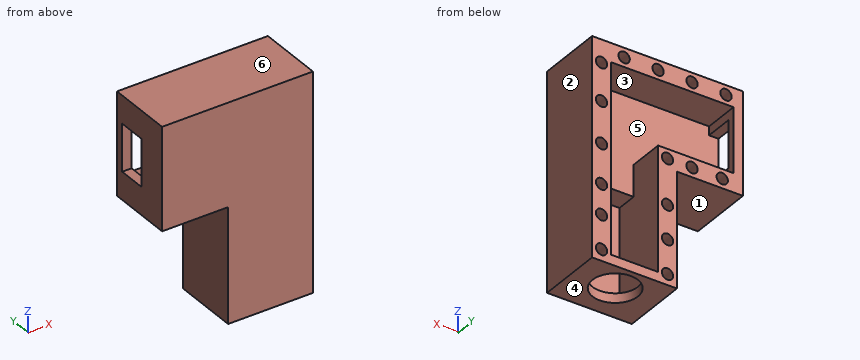
```python
from build123d import *

# Parameters (mm, degrees)
EXTRUDE_1_DEPTH     = 35
EXTRUDE_2_DEPTH     = 5
SKETCH_4_R          = 3
CUT_EXTRUDE_1_DEPTH = 20
SKETCH_6_W          = 25
SKETCH_6_H          = 16.678910785
EXTRUDE_3_DEPTH     = 11
SKETCH_7_W          = 65
SKETCH_7_H          = 34.285714286
EXTRUDE_4_DEPTH     = 11
SKETCH_8_R          = 12.052464441
CUT_EXTRUDE_2_DEPTH = 11
SKETCH_9_W          = 25
SKETCH_9_H          = 15
CUT_EXTRUDE_3_DEPTH = 11


with BuildPart() as part:
    # Эскиз1 → Бобышка-Вытянуть1 (new body)
    with BuildSketch(Plane(origin=(0, 0, 0), x_dir=(1, 0, 0), z_dir=(0, 1, 0))):
        Polygon((-25.991917961, 25.824175824), (0, 25.824175824), (0, 86.538461538), (45, 86.538461538), (45, -28.461538462), (-35, -28.461538462), (-35, 25.824175824), align=None)
        Polygon((-30, -18.461538462), (35, -18.461538462), (35, 21.538461538), (35, 81.538461538), (10, 81.538461538), (10, 15.824175824), (-30, 15.824175824), align=None, mode=Mode.SUBTRACT)
    extrude(amount=EXTRUDE_1_DEPTH)

    # Эскиз3 → Бобышка-Вытянуть2 (add)
    with BuildSketch(Plane.XZ):
        Polygon((35, -81.538461538), (35, 18.461538462), (-30, 18.461538462), (-30, -15.824175824), (10, -15.824175824), (10, -81.538461538), align=None)
    extrude(amount=-EXTRUDE_2_DEPTH)

    # Эскиз4 → Вырез-Вытянуть1 (cut)
    with BuildSketch(Plane(origin=(0, 35, 0), x_dir=(1, 0, 0), z_dir=(0, 1, 0))):
        with Locations(Location((40, 80.538461538, 0), (0, 0, 270))):
            Circle(SKETCH_4_R)
        with Locations(Location((40, 62.538461538, 0), (0, 0, 270))):
            Circle(SKETCH_4_R)
        with Locations(Location((40, 46.538461538, 0), (0, 0, 270))):
            Circle(SKETCH_4_R)
        with Locations(Location((40, 25.538461538, 0), (0, 0, 270))):
            Circle(SKETCH_4_R)
        with Locations(Location((40, 3.538461538, 0), (0, 0, 270))):
            Circle(SKETCH_4_R)
        with Locations(Location((40, -16.461538462, 0), (0, 0, 270))):
            Circle(SKETCH_4_R)
        with Locations(Location((5, 80.824175824, 0), (0, 0, 270))):
            Circle(SKETCH_4_R)
        with Locations(Location((5, 62.824175824, 0), (0, 0, 270))):
            Circle(SKETCH_4_R)
        with Locations(Location((5, 44.824175824, 0), (0, 0, 270))):
            Circle(SKETCH_4_R)
        with Locations(Location((-24, 20.824175824, 0), (0, 0, 270))):
            Circle(SKETCH_4_R)
        with Locations(Location((-8, 20.824175824, 0), (0, 0, 270))):
            Circle(SKETCH_4_R)
        with Locations(Location((5, 20.824175824, 0), (0, 0, 270))):
            Circle(SKETCH_4_R)
        with Locations(Location((-26, -23.461538462, 0), (0, 0, 270))):
            Circle(SKETCH_4_R)
        with Locations(Location((-8, -23.461538462, 0), (0, 0, 270))):
            Circle(SKETCH_4_R)
        with Locations(Location((10, -23.461538462, 0), (0, 0, 270))):
            Circle(SKETCH_4_R)
        with Locations(Location((28, -23.461538462, 0), (0, 0, 270))):
            Circle(SKETCH_4_R)
    extrude(amount=-CUT_EXTRUDE_1_DEPTH, mode=Mode.SUBTRACT)

    # Эскиз6 → Бобышка-Вытянуть3 (add)
    with BuildSketch(Plane(origin=(0, 5, 0), x_dir=(1, 0, 0), z_dir=(0, 1, 0))):
        with Locations((22.5, 24.163631217)):
            Rectangle(SKETCH_6_W, SKETCH_6_H)
    extrude(amount=EXTRUDE_3_DEPTH)

    # Эскиз7 → Бобышка-Вытянуть4 (add)
    with BuildSketch(Plane(origin=(0, 5, 0), x_dir=(1, 0, 0), z_dir=(0, 1, 0))):
        with Locations((2.5, -1.318681319)):
            Rectangle(SKETCH_7_W, SKETCH_7_H)
    extrude(amount=EXTRUDE_4_DEPTH)

    # Эскиз8 → Вырез-Вытянуть2 (cut)
    with BuildSketch(Plane.XY.offset(-81.538461538)):
        with Locations((22.5, 20)):
            Circle(SKETCH_8_R)
    extrude(amount=-CUT_EXTRUDE_2_DEPTH, mode=Mode.SUBTRACT)

    # Эскиз9 → Вырез-Вытянуть3 (cut)
    with BuildSketch(Plane(origin=(-30, 0, 0), x_dir=(0, 0, -1), z_dir=(1, 0, 0))):
        with Locations((-1.318681319, 23.5)):
            Rectangle(SKETCH_9_W, SKETCH_9_H)
    extrude(amount=-CUT_EXTRUDE_3_DEPTH, mode=Mode.SUBTRACT)


solid = part.part
```
Here's how the part is built. I have some questions about the finished solid (model axes, mm). Face numbers are marked on the shaded views. A direction names the side the tool comes from. Give positions to 0.01 mm unless a question says otherwise; leave off trailing zeros. Order: outer loops, then holes, each group sorted by start corner. A loop starts at its lowest first (then second) coordinate and runs counter-clockwise, first axis right, second up. Notation, with made-up numbers: (39, -7.5) - (86, -7.5) arc R30 cw to (86, 25.5) - close; hole circle Ø9 at (-28.5, -29). An arc over 180 degrees is marked (long way). Answer as a JSON object with one key per item and string values. Group by question number.
Item 1: For P1, Ø5.5, axis at x = -26, z = 23.46, coming from the +Y side; P2, Ø5, axis at x = -26, y = 22, coming from the -Z side, each with a flat end and sliding along its axis, tell me the tip position at first contact or that it passes through.
Item 2: If we section it at B-B on z = -13.5: Please give me the cut outline in (x, y).
Item 3: If we section it at D-D on x = -8: Please give me the cut outline in (y, z), and give its area (3 significant figures).
Item 4: Which directions (+Z, -Z, +X, -X, +Y, -Y) give clear straight access to the entire face, cutting with the end or side of a thin tool? Please do the marked faces 1, 2 and 3.
Item 5: Please list where these lines run through material, in increasing order: probe 1 along X at (y, z) = (26, -74.5); probe 2 along Z at (x, y) = (-18, 12); probe 3 along Z at (x, y) = (15.5, 22).
Item 6: If we section it at A-A on x = 22.5: Please give me the cut outline in (y, z), and give its area (3 significant figures).
Item 7: If we mould it in two halves opening along Z, with no side actions, what happens to the marked faces 4, 5 and 6? For each: pulls with the +Z half, pulls with the -Z half, needs draft (parallel to the pull), parting line crosses it, or undercut.
Item 8: If we section it at C-C on y = 20: Give the number of separate pieces and of enclosed holes in the cut face, and give its area (3 significant figures).
Result set:
{
 "1": {"P1": "y = 15", "P2": "z = -25.82"},
 "2": {"outline": "(-35, 0) - (45, 0) - (45, 35) - (35, 35) - (35, 16) - (-30, 16) - (-30, 35) - (-35, 35) - close"},
 "3": {"outline": "(0, -25.82) - (35, -25.82) - (35, -23.82) - (15, -23.82) - (15, -17.82) - (35, -17.82) - (35, -15.82) - (16, -15.82) - (16, 18.46) - (35, 18.46) - (35, 20.46) - (15, 20.46) - (15, 26.46) - (35, 26.46) - (35, 28.46) - (0, 28.46) - close", "area": "1,010 mm²"},
 "4": {"face 1": "-Z, -X, +Y, -Y", "face 2": "+Z, -Z, +X, +Y, -Y", "face 3": "+Y"},
 "5": {"probe 1": "0 to 10, 35 to 45", "probe 2": "-25.82 to 28.46", "probe 3": "18.46 to 28.46"},
 "6": {"outline": "(0, -86.54) - (7.95, -86.54) - (7.95, -81.54) - (5, -81.54) - (5, -32.5) - (16, -32.5) - (16, 18.46) - (35, 18.46) - (35, 28.46) - (0, 28.46) - close; (32.05, -86.54) - (35, -86.54) - (35, -81.54) - (32.05, -81.54) - close", "area": "1,470 mm²"},
 "7": {"face 4": "pulls with the -Z half", "face 5": "undercut", "face 6": "pulls with the +Z half"},
 "8": {"separate pieces": "2", "enclosed holes": "16", "area": "2,510 mm²"}
}
